```python
from build123d import *

# Parameters (mm, degrees)
SKETCH_1_W                 = 42
SKETCH_1_H                 = 35
EXTRUDE_1_DEPTH            = 10
SKETCH_2_W                 = 6.5
SKETCH_2_H                 = 21
CUT_EXTRUDE_1_DEPTH        = 10
SKETCH_5_W                 = 9
SKETCH_5_H                 = 11.5
EXTRUDE_2_DEPTH            = 10
SKETCH_6_R                 = 1.4
CUT_EXTRUDE_4_DEPTH        = 10
SKETCH_3_W                 = 44
SKETCH_3_H                 = 8
CUT_EXTRUDE_2_DEPTH        = 6
CUT_EXTRUDE_1_2_DEPTH      = 37.142080737
CUT_EXTRUDE_1_2_DEPTH_BACK = 10
SKETCH_8_W                 = 59.417014287
SKETCH_8_H                 = 10
EXTRUDE_3_DEPTH            = 3.5
SKETCH_12_W                = 60
SKETCH_12_H                = 23.5
CUT_EXTRUDE_5_DEPTH        = 8
FILLET_1_R                 = 5
FILLET_3_R                 = 2
CHAMFER_1_SIZE             = 4


with BuildPart() as part:
    # 草图1 → 凸台-拉伸1 (new body)
    with BuildSketch(Plane.XY):
        Rectangle(SKETCH_1_W, SKETCH_1_H)
    extrude(amount=EXTRUDE_1_DEPTH)

    # 草图2 → Cut-Extrude 1 (cut)
    with BuildSketch(Plane.XY.offset(10)):
        with Locations((-9.75, -2.5)):
            Rectangle(SKETCH_2_W, SKETCH_2_H)
        with Locations((9.75, -2.5)):
            Rectangle(SKETCH_2_W, SKETCH_2_H)
    extrude(amount=-CUT_EXTRUDE_1_DEPTH, mode=Mode.SUBTRACT)

    # 草图5 → 凸台-拉伸2 (add)
    with BuildSketch(Plane(origin=(0, 0, 0), x_dir=(-1, 0, 0), z_dir=(0, 0, -1))):
        with Locations((-25.5, 11.75)):
            Rectangle(SKETCH_5_W, SKETCH_5_H)
        with Locations((25.5, 11.75)):
            Rectangle(SKETCH_5_W, SKETCH_5_H)
    extrude(amount=-EXTRUDE_2_DEPTH)

    # 草图6 → 切除-拉伸4 (cut)
    with BuildSketch(Plane(origin=(0, 0, 0), x_dir=(-1, 0, 0), z_dir=(0, 0, -1))):
        with Locations((-25.1, 14.5)):
            Circle(SKETCH_6_R)
        with Locations((25.1, 14.5)):
            Circle(SKETCH_6_R)
        with Locations((-15.2, -9.1)):
            Circle(SKETCH_6_R)
        with Locations((15.2, -9.1)):
            Circle(SKETCH_6_R)
    extrude(amount=-CUT_EXTRUDE_4_DEPTH, mode=Mode.SUBTRACT)

    # 草图3 → 切除-拉伸2 (cut)
    with BuildSketch(Plane(origin=(0, 0, 0), x_dir=(-1, 0, 0), z_dir=(0, 0, -1))):
        with Locations((0, 13.5)):
            Rectangle(SKETCH_3_W, SKETCH_3_H)
    extrude(amount=-CUT_EXTRUDE_2_DEPTH, mode=Mode.SUBTRACT)

    # 草图8 → Cut-Extrude 1 2 (cut, two sides: drawn at the far end of the back side and taken through both)
    with BuildSketch(Plane.XY.offset(10).offset(-CUT_EXTRUDE_1_2_DEPTH_BACK)):
        with Locations((3.029489766, -20.5)):
            Rectangle(SKETCH_8_W, SKETCH_8_H)
    extrude(amount=CUT_EXTRUDE_1_2_DEPTH + CUT_EXTRUDE_1_2_DEPTH_BACK, mode=Mode.SUBTRACT)

    # 草图10 → 凸台-拉伸3 (add)
    with BuildSketch(Plane(origin=(0, 0, 0), x_dir=(-1, 0, 0), z_dir=(0, 0, -1))):
        Polygon((-28, 17.5), (-30, 17.5), (-30, 6), (-21, 6), (-21, -15.5), (0, -15.5), (0, -13.5), (-19, -13.5), (-19, 7), (-28, 7), align=None)
        Polygon((0, -13.5), (0, -15.5), (21, -15.5), (21, 6), (30, 6), (30, 17.5), (28, 17.5), (28, 7), (19, 7), (19, -13.5), align=None)
    extrude(amount=EXTRUDE_3_DEPTH)

    # 草图12 → 切除-拉伸5 (cut)
    with BuildSketch(Plane.XY.offset(10)):
        with Locations((0, -3.75)):
            Rectangle(SKETCH_12_W, SKETCH_12_H)
    extrude(amount=-CUT_EXTRUDE_5_DEPTH, mode=Mode.SUBTRACT)

    # 圆角1
    fillet_1_edges = [part.edges().sort_by_distance(p)[0] for p in [
        (-21, 6, -0.75),
        (21, 6, -0.75),
    ]]
    fillet(fillet_1_edges, radius=FILLET_1_R)

    # 圆角3
    fillet_3_edges = [part.edges().sort_by_distance(p)[0] for p in [
        (21.5, 8, 2),
        (-21.5, 8, 2),
        (0, 8, 2),
    ]]
    fillet(fillet_3_edges, radius=FILLET_3_R - 0.0001)  # a hair under: the kernel refuses the full size

    # 倒角1
    chamfer_1_edges = [part.edges().sort_by_distance(p)[0] for p in [
        (0, 8, 10),
    ]]
    chamfer(chamfer_1_edges, length=CHAMFER_1_SIZE)


solid = part.part
```
Input: part model. Units: mm. Frame: model coordinates. A direction names the side the tool comes from. Round coordinates to 2 decimals unless told otherwise and drop trailing zeros. Loops run counter-clockwise (first coordinate to the right, second up) from the corner with the lowest first, then second, coordinate; pieces in that order, holes last. Notation, with made-up numbers: (64.5, 84.25) - (118.5, 84.25) arc R24 ccw to (118.5, 105.25) - close; hole circle Ø1 at (-25.75, 87.5). An arc over 180 degrees is marked (long way). One line per item, written item: value. Start each with the question number.
(1) Section B-B, the plane x = -9. Return loops of the section in (y, z), plus the area to 3 significant figures.
(2) Contact query for flat-ended pins moving along their axis: P1, Ø3, axis at y = -5.5, z = -0.5, coming from the +X side; P2, Ø4, axis at x = -15.5, y = 2.5, coming from the -Z side; P3, Ø2, axis at x = -25.1, y = 14.5, coming from the -Z side; P4, Ø5, axis at x = 8.5, y = -5, coming from the +Z side. Output: stop coordinate, or through.
(3) Access query for faces 1 (the flat face through (13, -3, 1)), 2 (the flat face through (0, -5, 2)), 3 (the flat face through (-28, 12, -2)). Directions: +Z, -Z, +X, -X, +Y, -Y. A direction counts if a zero-diameter tool reaches every point of the face in a straight line with its end or side. Return the directions, or none.
(4) Ray query, line 1 (X direction, y = -1.5, z = 0.5); line 2 (X direction, y = 11.5, z = -0.5); line 3 (Y direction, x = 25.1, z = 4.5). Return the intervals inside material, ascending. Write a range as [from, to].
(5) Section D-D, the plane z = 3. Return loops of the section in (x, y), plus the area to 3 significant figures.
(6) Draft query along X for faces 4 (the flat face through (-21, -7, -1)), 5 (the flat face through (-28, 6, -1)), 6 (the cylindrical face through (24.35, 15.68, 4.93)). Return one class per face: +X half, -X half, draft (parallel to the pull), parting line (faces both ways), or undercut.
(7) Section C-C, the plane y = -9.1. Return loops of the section in (x, z).
(8) Section A-A, the plane y = 14.5. Return loops of the section in (x, z).
Results below:
1. outline: (-15.5, -3.5) - (-13.5, -3.5) - (-13.5, 0) - (-13, 0) - (-13, 2) - (-15.5, 2) - close; (8, 0) - (9.5, 0) - (9.5, 6) - (17.5, 6) - (17.5, 10) - (12, 10) - (8, 6) - close
1. area: 51.0 mm^2
2. P1: x = 21
2. P2: z = 0
2. P3: through
2. P4: z = 2
3. face 1: +Z, -Z
3. face 2: +Z, +X, -X, -Y
3. face 3: -Z, +Y
4. line 1: [-21, -13], [-6.5, 6.5], [13, 21]
4. line 2: [-30, -28], [28, 30]
4. line 3: [8, 13.1], [15.9, 17.5]
5. outline: (-30, 7.73) - (-13, 7.73) - (-13, 8) - (-6.5, 8) - (-6.5, 7.73) - (6.5, 7.73) - (6.5, 8) - (13, 8) - (13, 7.73) - (30, 7.73) - (30, 17.5) - (22, 17.5) - (22, 9.5) - (-22, 9.5) - (-22, 17.5) - (-30, 17.5) - close; hole circle Ø2.8 at (-25.1, 14.5); hole circle Ø2.8 at (25.1, 14.5)
5. area: 218 mm^2
6. face 4: -X half
6. face 5: draft
6. face 6: undercut
7. outline: (-21, -3.5) - (-19, -3.5) - (-19, 0) - (-16.6, 0) - (-16.6, 2) - (-21, 2) - close; (-13.8, 0) - (-13, 0) - (-13, 2) - (-13.8, 2) - close; (-6.5, 0) - (6.5, 0) - (6.5, 2) - (-6.5, 2) - close; (13, 0) - (13.8, 0) - (13.8, 2) - (13, 2) - close; (16.6, 0) - (19, 0) - (19, -3.5) - (21, -3.5) - (21, 2) - (16.6, 2) - close
8. outline: (-30, -3.5) - (-28, -3.5) - (-28, 0) - (-26.5, 0) - (-26.5, 10) - (-30, 10) - close; (-23.7, 0) - (-22, 0) - (-22, 6) - (22, 6) - (22, 0) - (23.7, 0) - (23.7, 10) - (-23.7, 10) - close; (26.5, 0) - (28, 0) - (28, -3.5) - (30, -3.5) - (30, 10) - (26.5, 10) - close
